Input: part model. Units: mm. Frame: model coordinates. Face numbers are marked on the shaded views. A direction names the side the tool comes from. Coordinates: 2 decimals unless noted, no trailing zeros. Write each loop counter-clockwise with the first axis right and the second up, starting at its lowest first coordinate (ties: lowest second). Pieces come first, ordered by that corner, then holes. Notation, with made-up numbers: (18.25, 8.5) - (62.25, 8.5) arc R18 ccw to (62.25, 36.5) - close; hole circle Ø4 at (-31.5, 60.5). An arc over 180 degrees is marked (long way). Use CSV: the item, a comma, the result in double quotes.
```python
from build123d import *

# Parameters (mm, degrees)
SKETCH1_W           = 88
SKETCH1_H           = 40
BOSS_EXTRUDE1_DEPTH = 100
SKETCH2_R           = 5.5
CUT_EXTRUDE1_DEPTH  = 40
CUT_EXTRUDE2_START  = -13.73686
SKETCH3_R           = 2.75
CUT_EXTRUDE2_DEPTH  = 13.73686
SKETCH5_R           = 2.75
CUT_EXTRUDE3_DEPTH  = 3
SKETCH6_R           = 2.75
CUT_EXTRUDE4_DEPTH  = 3
SKETCH7_R           = 7.5
SKETCH7_R_2         = 3.25
BOSS_EXTRUDE2_DEPTH = 1
SKETCH8_R           = 7.5
SKETCH8_R_2         = 3.25
BOSS_EXTRUDE3_DEPTH = 1
SKETCH9_R           = 7
CUT_EXTRUDE5_DEPTH  = 1.5
SKETCH10_R          = 7
CUT_EXTRUDE6_DEPTH  = 1.5


with BuildPart() as part:
    # Sketch1 → Boss-Extrude1 (new body)
    with BuildSketch(Plane.XY):
        with Locations((44, 20)):
            Rectangle(SKETCH1_W, SKETCH1_H)
    extrude(amount=BOSS_EXTRUDE1_DEPTH)

    # Sketch2 → Cut-Extrude1 (cut)
    with BuildSketch(Plane.XZ):
        with Locations((44, 18.5)):
            Circle(SKETCH2_R)
        with BuildLine():
            Line((20, 3), (32, 3))
            ThreePointArc((32, 3), (32.353553391, 3.146446609), (32.5, 3.5))
            Line((32.5, 3.5), (32.5, 19))
            ThreePointArc((32.5, 19), (35.721825407, 26.778174593), (43.5, 30))
            Line((43.5, 30), (44.5, 30))
            ThreePointArc((44.5, 30), (52.278174593, 26.778174593), (55.5, 19))
            Line((55.5, 19), (55.5, 3.5))
            ThreePointArc((55.5, 3.5), (55.646446609, 3.146446609), (56, 3))
            Line((56, 3), (68, 3))
            ThreePointArc((68, 3), (80.02081528, 7.97918472), (85, 20))
            Line((85, 20), (85, 100))
            Line((85, 100), (3, 100))
            Line((3, 100), (3, 20))
            ThreePointArc((3, 20), (7.97918472, 7.97918472), (20, 3))
        make_face()
        with BuildLine():
            Line((0, 20), (0, 0))
            Line((0, 0), (20, 0))
            ThreePointArc((20, 0), (5.857864376, 5.857864376), (0, 20))
        make_face()
        with BuildLine():
            Line((68, 0), (88, 0))
            Line((88, 0), (88, 20))
            ThreePointArc((88, 20), (82.142135624, 5.857864376), (68, 0))
        make_face()
        with BuildLine():
            Line((40.5, 9), (47.5, 9))
            ThreePointArc((47.5, 9), (47.853553391, 8.853553391), (48, 8.5))
            Line((48, 8.5), (48, 4.5))
            ThreePointArc((48, 4.5), (47.853553391, 4.146446609), (47.5, 4))
            Line((47.5, 4), (40.5, 4))
            ThreePointArc((40.5, 4), (40.146446609, 4.146446609), (40, 4.5))
            Line((40, 4.5), (40, 8.5))
            ThreePointArc((40, 8.5), (40.146446609, 8.853553391), (40.5, 9))
        make_face()
    extrude(amount=-CUT_EXTRUDE1_DEPTH, mode=Mode.SUBTRACT)

    # Sketch3 → Cut-Extrude2 (cut)
    with BuildSketch(Plane(origin=(0, 0, 0), x_dir=(-1, 0, 0), z_dir=(0, 0, -1)).offset(CUT_EXTRUDE2_START)):
        with Locations((-44, 20)):
            Circle(SKETCH3_R)
    extrude(amount=CUT_EXTRUDE2_DEPTH, mode=Mode.SUBTRACT)

    # Sketch5 → Cut-Extrude3 (cut)
    with BuildSketch(Plane(origin=(88, 0, 0), x_dir=(0, 0, -1), z_dir=(1, 0, 0))):
        with Locations((-90, 20)):
            Circle(SKETCH5_R)
        with BuildLine():
            Line((-27, 0), (-100, 0))
            Line((-100, 0), (-100, 18.582255312))
            ThreePointArc((-100, 18.582255312), (-97.188609996, 12.905362143), (-91.549199975, 10.01952008))
            Line((-91.549199975, 10.01952008), (-27, 0))
        make_face()
        with BuildLine():
            Line((-100, 40), (-27, 40))
            Line((-27, 40), (-91.549199975, 29.98047992))
            ThreePointArc((-91.549199975, 29.98047992), (-97.188609996, 27.094637857), (-100, 21.417744688))
            Line((-100, 21.417744688), (-100, 40))
        make_face()
    extrude(amount=-CUT_EXTRUDE3_DEPTH, mode=Mode.SUBTRACT)

    # Sketch6 → Cut-Extrude4 (cut)
    with BuildSketch(Plane.ZY):
        with Locations((90, 20)):
            Circle(SKETCH6_R)
        with BuildLine():
            Line((100, 0), (100, 18.582255312))
            ThreePointArc((100, 18.582255312), (97.188609996, 12.905362143), (91.549199975, 10.01952008))
            Line((91.549199975, 10.01952008), (27, 0))
            Line((27, 0), (100, 0))
        make_face()
        with BuildLine():
            Line((100, 21.417744688), (100, 40))
            Line((100, 40), (27, 40))
            Line((27, 40), (91.549199975, 29.98047992))
            ThreePointArc((91.549199975, 29.98047992), (97.188609996, 27.094637857), (100, 21.417744688))
        make_face()
    extrude(amount=-CUT_EXTRUDE4_DEPTH, mode=Mode.SUBTRACT)

    # Sketch7 → Boss-Extrude2 (add)
    with BuildSketch(Plane(origin=(3, 0, 0), x_dir=(0, 0, -1), z_dir=(1, 0, 0))):
        with Locations((-90, 20)):
            Circle(SKETCH7_R)
        with Locations((-90, 20)):
            Circle(SKETCH7_R_2, mode=Mode.SUBTRACT)
    extrude(amount=BOSS_EXTRUDE2_DEPTH)

    # Sketch8 → Boss-Extrude3 (add)
    with BuildSketch(Plane.ZY.offset(-85)):
        with Locations((90, 20)):
            Circle(SKETCH8_R)
        with Locations((90, 20)):
            Circle(SKETCH8_R_2, mode=Mode.SUBTRACT)
    extrude(amount=BOSS_EXTRUDE3_DEPTH)

    # Sketch9 → Cut-Extrude5 (cut)
    with BuildSketch(Plane(origin=(88, 0, 0), x_dir=(0, 0, -1), z_dir=(1, 0, 0))):
        with Locations((-90, 20)):
            Circle(SKETCH9_R)
    extrude(amount=-CUT_EXTRUDE5_DEPTH, mode=Mode.SUBTRACT)

    # Sketch10 → Cut-Extrude6 (cut)
    with BuildSketch(Plane.ZY):
        with Locations((90, 20)):
            Circle(SKETCH10_R)
    extrude(amount=-CUT_EXTRUDE6_DEPTH, mode=Mode.SUBTRACT)


solid = part.part
```
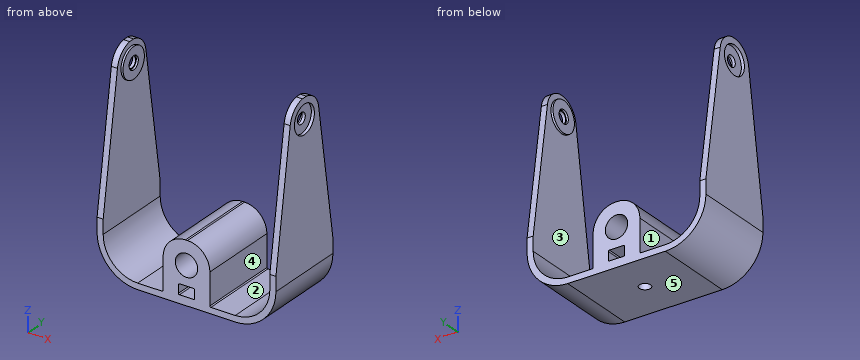
(1) Ray query, probe 1 along X at (y, z) = (29, 37); probe 2 along Y at (x, z) = (84.7, 90); probe 3 along X at (y, z) = (24, 22). Return the intervals inside material, ascending. Write a range as from..to.
Check values:
probe 1,"0..3, 85..88"
probe 2,"12.5..16.75, 23.25..27.5"
probe 3,"0..3, 32.92..39.76, 48.24..55.08, 85..88"
(2) Cut plane A-A on z = 45. Return loops of the section in (x, y), and give its area (3 significant figures).
Check values:
outline,"(0, 2.79) - (3, 2.79) - (3, 37.21) - (0, 37.21) - close; (85, 2.79) - (88, 2.79) - (88, 37.21) - (85, 37.21) - close"
area,"206 mm^2"
(3) Pin query (flat end, axial travel): pin 1 Ø4.5 at (y, z) = (19.5, 92) entering from +X; pin 2 Ø5 at (x, y) = (44, 20) entering from -Z; pin 3 Ø3.5 at (x, y) = (45, 15) entering from +Z. Return the tip coordinate at first contact, or that it passes through.
Check values:
pin 1,"x = 86.5"
pin 2,"z = 23.4"
pin 3,"z = 30"
(4) Reachability of the marked faces 4 and 5 from +Z, -Z, +X, -X, +Y, -Y: full face, straight path, thin tool, end or side. Return the list, or none.
Check values:
face 4,"+Z, +Y, -Y"
face 5,"-Z, +X, -X, +Y, -Y"
(5) Cut plane D-D on x = 63.5. Return loops of the section in (y, z).
Check values:
outline,"(0, 0) - (40, 0) - (40, 3) - (0, 3) - close"
(6) Cut plane B-B on y = 6.5. State how many separate pieces and enclosed holes the cut face has, and give its area (3 significant figures).
Check values:
separate pieces,"1"
enclosed holes,"2"
area,"1,050 mm^2"
(7) Draft query along Z for the marked faces 1, 2 and 3. Return one class per face: pulls with the +Z half, pulls with the -Z half, needs draft (parallel to the pull), parting line crosses it, or undercut.
Check values:
face 1,"needs draft"
face 2,"pulls with the +Z half"
face 3,"undercut"
